```python
from build123d import *

# Parameters (mm, degrees)
SKETCH_1_W                  = 86
SKETCH_1_H                  = 44.2
EXTRUDE_1_DEPTH             = 14.2
EXTRUDE_2_DEPTH             = 5
SKETCH_3_W                  = 81.1
SKETCH_3_H                  = 42.4
CUT_EXTRUDE_1_DEPTH         = 18.3
HOLE_WIZARD_8_3_8_3_1_D     = 8.3
HOLE_WIZARD_8_3_8_3_1_DEPTH = 3.2
FILLET_1_R                  = 3
FILLET_2_R                  = 3
FILLET_3_R                  = 3
FILLET_4_R                  = 3
FILLET_5_R                  = 3
EXTRUDE_START               = -3
SKETCH_6_R                  = 4.15
EXTRUDE_3_DEPTH             = 3


with BuildPart() as part:
    # Эскиз1 → Бобышка-Вытянуть1 (new body)
    with BuildSketch(Plane.XY.offset(9.6)):
        with Locations((47, 0)):
            Rectangle(SKETCH_1_W, SKETCH_1_H)
    extrude(amount=-EXTRUDE_1_DEPTH)

    # Эскиз2 → Бобышка-Вытянуть2 (add)
    with BuildSketch(Plane(origin=(0, 0, -4.6), x_dir=(-1, 0, 0), z_dir=(0, 0, -1))):
        with BuildLine():
            Line((-90, -22.1), (-90, -17.1))
            ThreePointArc((-90, -17.1), (-104, 0), (-90, 17.1))
            Line((-90, 17.1), (-90, 22.1))
            Line((-90, 22.1), (-4, 22.1))
            Line((-4, 22.1), (-4, -22.1))
            Line((-4, -22.1), (-90, -22.1))
        make_face()
        with BuildLine():
            Line((-90, -12.994779171), (-90, 12.994779171))
            ThreePointArc((-90, 12.994779171), (-100, 0), (-90, -12.994779171))
        make_face(mode=Mode.SUBTRACT)
    extrude(amount=EXTRUDE_2_DEPTH)

    # Эскиз3 → Вырез-Вытянуть1 (cut)
    with BuildSketch(Plane.XY.offset(9.6)):
        with Locations((48.55, 0)):
            Rectangle(SKETCH_3_W, SKETCH_3_H)
    extrude(amount=-CUT_EXTRUDE_1_DEPTH, mode=Mode.SUBTRACT)

    # Диаметр отверстия Ø8.3 (8.3)1
    with Locations(Plane.ZY.offset(-4)):
        with Locations((0, 0)):
            Hole(HOLE_WIZARD_8_3_8_3_1_D / 2, depth=HOLE_WIZARD_8_3_8_3_1_DEPTH)

    # Скругление1
    fillet_1_edges = [part.edges().sort_by_distance(p)[0] for p in [
        (4, -22.1, 0),
        (4, 22.1, 0),
    ]]
    fillet(fillet_1_edges, radius=FILLET_1_R)

    # Скругление2
    fillet_2_edges = [part.edges().sort_by_distance(p)[0] for p in [
        (48.55, -21.2, -8.7),
    ]]
    fillet(fillet_2_edges, radius=FILLET_2_R)

    # Скругление3
    fillet_3_edges = [part.edges().sort_by_distance(p)[0] for p in [
        (48.55, 21.2, -8.7),
    ]]
    fillet(fillet_3_edges, radius=FILLET_3_R)

    # Скругление4
    fillet_4_edges = [part.edges().sort_by_distance(p)[0] for p in [
        (8, -21.2, 1.95),
        (8, -20.321320344, -7.821320344),
        (8, 0, -8.7),
        (8, 21.2, 1.95),
        (8, 20.321320344, -7.821320344),
    ]]
    fillet(fillet_4_edges, radius=FILLET_4_R)

    # Скругление5
    fillet_5_edges = [part.edges().sort_by_distance(p)[0] for p in [
        (89.1, -21.2, 1.95),
        (89.1, 0, -8.7),
        (89.1, -20.321320344, -7.821320344),
        (89.1, 21.2, 1.95),
        (89.1, 20.321320344, -7.821320344),
    ]]
    fillet(fillet_5_edges, radius=FILLET_5_R)

    # Эскиз6 → Бобышка-Вытянуть3 (add)
    with BuildSketch(Plane.ZY.offset(-4).offset(EXTRUDE_START)):
        Circle(SKETCH_6_R)
    extrude(amount=EXTRUDE_3_DEPTH)


solid = part.part
```
Could you check a few things on this model? Use its own coordinates, in mm. A direction names the side the tool comes from. Give positions to 0.01 mm unless a question says otherwise; leave off trailing zeros. Write each loop counter-clockwise with the first axis right and the second up, starting at its lowest first coordinate (ties: lowest second). Pieces come first, ordered by that corner, then holes. Notation, with made-up numbers: (-14, -7.5) -> (11, -7.5) arc R18 ccw to (11, 27.5) -> close; hole circle Ø10 at (55.5, 46.5). An arc over 180 degrees is marked (long way). Write each question's results on one line, items separated by ' | '.
1. On a 3-axis mill with a long thin cutter (end or side, diameter ignored), from which of +Z, -Z, +X, -X, +Y, -Y can I reach the whole of each face in a straight line? I mean faces 1 (the cylindrical face through (4.9, -21.24, -0.13)), 2 (the flat face through (100.1, 1.3, -4.6)), 3 (the cylindrical face through (8.86, 0.25, -7.8)), 4 (the cylindrical face through (104, 0, -7)), 5 (the flat face through (7.2, 0, 0)). Say none if no direction works.
Check sheet entries:
face 1: +Z, -Z, -X, -Y | face 2: +Z, +X, +Y, -Y | face 3: +Z | face 4: +Z, -Z, +X | face 5: none
2. I want a section at B-B, the plane z = 8. Write out the boundary of the cut face in (x, y), then the cut area to 3 significant figures.
Check sheet entries:
outline: (4, -19.1) arc R3 ccw to (7, -22.1) -> (90, -22.1) -> (90, 22.1) -> (7, 22.1) arc R3 ccw to (4, 19.1) -> close; hole (8, -18.2) arc R3 ccw to (11, -21.2) -> (86.1, -21.2) arc R3 ccw to (89.1, -18.2) -> (89.1, 18.2) arc R3 ccw to (86.1, 21.2) -> (11, 21.2) arc R3 ccw to (8, 18.2) -> close | area: 366 mm²
3. If we mould it in two halves opening along X, with no side actions, what happens to faces 6 (the flat face through (48, -22.1, 0)), 7 (the cylindrical face through (88.2, 20.34, 2.06)), 8 (the cylindrical face through (4.9, 21.24, -0.13))? For each: released by +X, released by -X, zero draft, split by the parting line, or undercut.
Check sheet entries:
face 6: zero draft | face 7: undercut | face 8: released by -X
4. Will these pins go through, and if not, where does the flat tip stop? pin 1 Ø4.5 at (y, z) = (0.5, 0) entering from +X; pin 2 Ø1.5 at (x, y) = (94, -13) entering from +Z.
Check sheet entries:
pin 1: stops at x = 90 | pin 2: stops at z = -4.6
5. I want a section at A-A, the plane y = 0. Write out the boundary of the cut face in (x, z).
Check sheet entries:
outline: (4, -9.6) -> (90, -9.6) -> (90, 9.6) -> (89.1, 9.6) -> (89.1, -5.7) arc R3 cw to (86.1, -8.7) -> (11, -8.7) arc R3 cw to (8, -5.7) -> (8, 9.6) -> (4, 9.6) -> close; (100, -9.6) -> (104, -9.6) -> (104, -4.6) -> (100, -4.6) -> close; hole (7, -4.15) -> (7.2, -4.15) -> (7.2, 4.15) -> (7, 4.15) -> close
6. I need wall thicknesses on L1, parallel to Y at x = 51, z = -0.75; L2, parallel to X at y = -18, z = 3.25; L3, parallel to Y at x = 7.1, z = 0. Which ranges of each line are inside material? Lowest first, please.
Check sheet entries:
L1: y = -22.1 to -21.2, 21.2 to 22.1 | L2: x = 4 to 8, 89.1 to 90 | L3: y = -22.1 to -4.15, 4.15 to 22.1
7. I want a section at D-D, the plane x = 98.5. Write out the boundary of the cut face in (y, z), then the cut area to 3 significant figures.
Check sheet entries:
outline: (-12.71, -9.6) -> (-6.17, -9.6) -> (-6.17, -4.6) -> (-12.71, -4.6) -> close; (6.17, -9.6) -> (12.71, -9.6) -> (12.71, -4.6) -> (6.17, -4.6) -> close | area: 65.4 mm²
8. I want a section at C-C, the plane z = 0. Write out the boundary of the cut face in (x, y), then the cut area to 3 significant figures.
Check sheet entries:
outline: (4, -19.1) arc R3 ccw to (7, -22.1) -> (90, -22.1) -> (90, 22.1) -> (7, 22.1) arc R3 ccw to (4, 19.1) -> close; hole (7, -4.15) -> (7.2, -4.15) -> (7.2, 4.15) -> (7, 4.15) -> close; hole (8, -18.2) arc R3 ccw to (11, -21.2) -> (86.1, -21.2) arc R3 ccw to (89.1, -18.2) -> (89.1, 18.2) arc R3 ccw to (86.1, 21.2) -> (11, 21.2) arc R3 ccw to (8, 18.2) -> close | area: 365 mm²
